The model under review builds one solid part; all positions refer to its coordinate system, in mm. Face numbers are marked on the shaded views. A direction names the side the tool comes from. Coordinates: 2 decimals unless noted, no trailing zeros. Order: outer loops, then holes, each group sorted by start corner. A loop starts at its lowest first (then second) coordinate and runs counter-clockwise, first axis right, second up. Notation, with made-up numbers: (-15.5, 8) -> (19.5, 8) arc R18 ccw to (19.5, 18) -> close; hole circle Ø10 at (22.25, 80.5). An arc over 180 degrees is marked (long way). Put each result on its own line as item: value.
from build123d import *

# Parameters (mm, degrees)
F1_DEPTH = 127
F0_W     = 25.4
F0_H     = 19.05
F2_DEPTH = 25.4
F3_DEPTH = 7.9375
F5_R     = 6.35


with BuildPart() as f1:
    # F0 (on Front) → F1 (new body)
    with BuildSketch(Plane.XZ):
        Polygon((41.275, -9.525), (41.275, 9.525), (22.225, 9.525), (-41.275, 9.525), (-41.275, -9.525), align=None)
    extrude(amount=F1_DEPTH)

    # F0 (on Front) → F2 (join, symmetric)
    with BuildSketch(Plane.XZ):
        with BuildLine():
            Line((22.225, 9.525), (41.275, 9.525))
            Line((41.275, 9.525), (41.275, 31.3365191218))
            ThreePointArc((41.275, 31.3365191218), (45.0038822026, 39.8471765228), (53.788352915, 42.8752))
            Line((53.788352915, 42.8752), (60.325, 42.8752))
            Line((60.325, 42.8752), (60.325, 61.9252))
            Line((60.325, 61.9252), (54.3759968817, 61.9252))
            add(Edge.make_bspline(
                [(51.370796581, 61.9273374506), (52.3872818236, 61.9429580973), (53.3895331595, 61.9423398279), (54.3759968817, 61.9252)],
                knots=[106.1406160735, 106.1406160735, 106.1406160735, 106.1406160735, 109.0637160769, 109.0637160769, 109.0637160769, 109.0637160769], degree=3))
            ThreePointArc((51.370796581, 61.9273374506), (30.6779581359, 52.4627801751), (22.225, 31.3365191218))
            Line((22.225, 31.3365191218), (22.225, 9.525))
        make_face()
        with Locations((73.025, 52.4002)):
            Rectangle(F0_W, F0_H)
    extrude(amount=F2_DEPTH, both=True)

    # F0 (on Front) → F3 (join, symmetric)
    with BuildSketch(Plane.XZ):
        with BuildLine():
            Line((-41.275, 9.525), (22.225, 9.525))
            Line((22.225, 9.525), (22.225, 31.3365191218))
            ThreePointArc((22.225, 31.3365191218), (30.6779581359, 52.4627801751), (51.370796581, 61.9273374506))
            add(Edge.make_bspline(
                [(-41.275, 9.525), (-41.2155685722, 39.382135411), (14.4612246374, 61.3601365133), (51.370796581, 61.9273374506)],
                knots=[0, 0, 0, 0, 106.1406160735, 106.1406160735, 106.1406160735, 106.1406160735], degree=3))
        make_face()
    extrude(amount=F3_DEPTH, both=True)

    # F0 (on Front) → F4 (revolve)
    with BuildSketch(Plane.XZ):
        Polygon((85.725, 61.9252), (85.725, 42.8752), (85.725, 38.1), (111.125, 38.1), (111.125, 66.675), (85.725, 66.675), align=None)
    revolve(axis=Axis((85.725, 0, 52.3875), (0, 0, 1)))

    # F5
    f5_edges = [f1.edges().sort_by_distance(p)[0] for p in [
        (41.275, -127, 0),
        (-41.275, -127, 0),
        (41.275, 0, 0),
        (-41.275, 0, 0),
    ]]
    fillet(f5_edges, radius=F5_R)


solid = f1.part
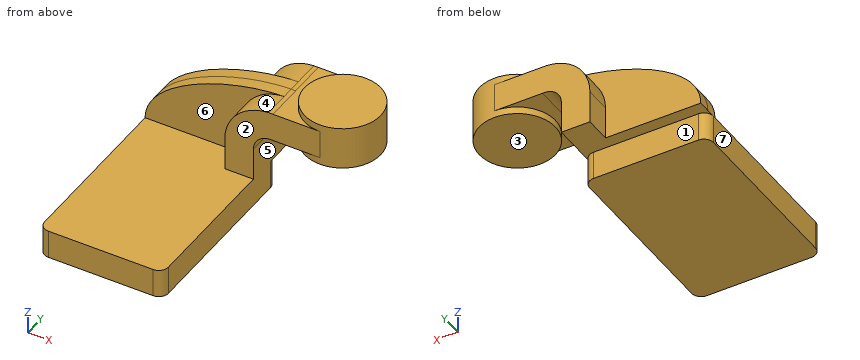
Item 1: For the marked faces 1, 2, 3 and 4, list the 3-axis set-ups (+Z, -Z, +X, -X, +Y, -Y) from which the entire face can be reached by the end or side of a thin tool; tool diameter is ignored.
Answers below:
face 1: -Z, +X, -X, +Y
face 2: +Z, +X, -X, -Y
face 3: -Z, +X, +Y, -Y
face 4: +Z, -X, -Y
Item 2: For pin 1 Ø5 at (y, z) = (19, 20.5) entering from -X (3 decimals); pin 2 Ø5 at (x, z) = (-7, 18.5) entering from -Y; pin 3 Ø15 at (x, z) = (-16, 2.5) entering from +Y, all flat-tipped, find the tip position at first contact; note any pin that passes through.
Answers below:
pin 1: x = 22.225
pin 2: y = -7.94
pin 3: y = 7.94
Item 3: Consider section C-C on y = -63.5. Write out the cut boundary in (x, z) (3 decimals).
Answers below:
outline: (-41.275, -9.525) -> (41.275, -9.525) -> (41.275, 9.525) -> (-41.275, 9.525) -> close
Item 4: Consider section A-A on x = 74. Write out the cut boundary in (y, z) (3 decimals), and give its area (3 significant figures).
Answers below:
outline: (-25.4, 42.875) -> (-22.532, 42.875) -> (-22.532, 38.1) -> (22.532, 38.1) -> (22.532, 42.875) -> (25.4, 42.875) -> (25.4, 61.925) -> (22.532, 61.925) -> (22.532, 66.675) -> (-22.532, 66.675) -> (-22.532, 61.925) -> (-25.4, 61.925) -> close
area: 1,400 mm^2
Item 5: Consider section B-B on z = 4. Write out the cut boundary in (x, y) (3 decimals), and give its area (3 significant figures).
Answers below:
outline: (-41.275, -120.65) arc R6.35 ccw to (-34.925, -127) -> (34.925, -127) arc R6.35 ccw to (41.275, -120.65) -> (41.275, -6.35) arc R6.35 ccw to (34.925, 0) -> (-34.925, 0) arc R6.35 ccw to (-41.275, -6.35) -> close
area: 10,400 mm^2
Item 6: For line 1 (Z direction, x = -4, y = -46) (3 decimals); line 2 (Y direction, x = 10, z = 42); line 3 (Y direction, x = 85, z = 60), list the stretches that pass through material, from the lowest coordinate up. Write a range as from..to.
Answers below:
line 1: -9.525..9.525
line 2: -7.94..7.94
line 3: -25.4..25.4
Item 7: Mouldability with a two-part tool opening along X and no side actions: class the marked faces 5, 6 and 7 as +X half, -X half, draft (parallel to the pull), parting line (faces both ways), or undercut.
Answers below:
face 5: +X half
face 6: draft
face 7: -X half
